```python
from build123d import *

# Parameters (mm, degrees)
SKETCH1_R           = 6.35
SKETCH1_R_2         = 4.699
BOSS_EXTRUDE1_DEPTH = 13.716
SKETCH2_R           = 7.5565
SKETCH2_R_2         = 6.096
BOSS_EXTRUDE2_DEPTH = 1.27
SKETCH3_R           = 6.35
BOSS_EXTRUDE3_DEPTH = 1.016


with BuildPart() as part:
    # Sketch1 → Boss-Extrude1 (new body)
    with BuildSketch(Plane(origin=(0, 0, 0), x_dir=(1, 0, 0), z_dir=(0, 1, 0))):
        Circle(SKETCH1_R)
        Circle(SKETCH1_R_2, mode=Mode.SUBTRACT)
    extrude(amount=BOSS_EXTRUDE1_DEPTH)

    # Sketch2 → Boss-Extrude2 (add)
    with BuildSketch(Plane(origin=(0, 0, 0), x_dir=(1, 0, 0), z_dir=(0, 1, 0))):
        Circle(SKETCH2_R)
        Circle(SKETCH2_R_2, mode=Mode.SUBTRACT)
    extrude(amount=BOSS_EXTRUDE2_DEPTH)

    # Sketch3 → Boss-Extrude3 (add)
    with BuildSketch(Plane(origin=(0, 13.716, 0), x_dir=(1, 0, 0), z_dir=(0, 1, 0))):
        Circle(SKETCH3_R)
    extrude(amount=-BOSS_EXTRUDE3_DEPTH)


solid = part.part
```
Verification items for the finished model (mm, model axes). A direction names the side the tool comes from. Give positions to 0.01 mm unless a question says otherwise; leave off trailing zeros. Order: outer loops, then holes, each group sorted by start corner. A loop starts at its lowest first (then second) coordinate and runs counter-clockwise, first axis right, second up. Notation, with made-up numbers: (46, -22.5) -> (66, -22.5) arc R16 ccw to (66, -4.5) -> close; hole circle Ø10 at (48.5, 8.5). An arc over 180 degrees is marked (long way). One line per item, written item: value.
(1) Gauge pin test, flat ends, axial feed: pin 1 (1.5 mm diameter, centred on x = -4.5, y = 8, fed in from +Z); pin 2 (5.5 mm diameter, centred on x = 0, z = 0, fed in from -Y); pin 3 (2 mm diameter, centred on y = 8.5, z = 1, fed in from +X). Record the tip position at first contact, or that the pin passes through.
Final values:
pin 1: z = 5.12
pin 2: y = 12.7
pin 3: x = 6.35
(2) Sectioned sample at D-D on x = 6. Record the cut outline in (y, z), then the cut area to 3 significant figures.
Final values:
outline: (0, -4.59) -> (1.27, -4.59) -> (1.27, -2.08) -> (13.72, -2.08) -> (13.72, 2.08) -> (1.27, 2.08) -> (1.27, 4.59) -> (0, 4.59) -> close
area: 63.4 mm^2
(3) Scan lines: line 1 along Z through (x, y) = (0, 4.25); line 2 along Y through (x, z) = (-3.25, 1.75). Record each from-to range of solid material in increasing order. Write a range as [from, to].
Final values:
line 1: [-6.35, -4.7], [4.7, 6.35]
line 2: [12.7, 13.72]
(4) Draft check along X on faces 1 (the face through (0, 13.716, 0)), 2 (the face through (0, 12.7, 0)), 3 (the face through (-0.61, 6.26, -4.66)), 4 (the face through (-5.569, 0.626, -5.107)). Enter one of: pulls with the +X half, pulls with the -X half, needs draft (parallel to the pull), parting line crosses it, or undercut.
Final values:
face 1: needs draft
face 2: undercut
face 3: undercut
face 4: parting line crosses it
(5) Sectioned sample at B-B on x = 0. Record the cut outline in (y, z), then the cut area to 3 significant figures.
Final values:
outline: (0, -7.56) -> (1.27, -7.56) -> (1.27, -6.35) -> (13.72, -6.35) -> (13.72, 6.35) -> (1.27, 6.35) -> (1.27, 7.56) -> (0, 7.56) -> (0, 4.7) -> (12.7, 4.7) -> (12.7, -4.7) -> (0, -4.7) -> close
area: 57.9 mm^2
(6) Tool access check on faces 5 (the face through (5, 0, 0)), 6 (the face through (-1.38, 7.41, 6.2)). Record the directions out of +Z, -Z, +X, -X, +Y, -Y that give a thin tool (end or side, any length) a straight path to the whole face; none if there is none.
Final values:
face 5: +Z, -Z, +X, -X, -Y
face 6: +Y
(7) Sectioned sample at C-C on y = 2.75. Record the cut outline in (x, z), then the cut area to 3 significant figures.
Final values:
outline: circle Ø12.7 at (0, 0); hole circle Ø9.4 at (0, 0)
area: 57.3 mm^2
(8) Sectioned sample at A-A on z = 0. Record the cut outline in (x, y).
Final values:
outline: (-7.56, 0) -> (-4.7, 0) -> (-4.7, 12.7) -> (4.7, 12.7) -> (4.7, 0) -> (7.56, 0) -> (7.56, 1.27) -> (6.35, 1.27) -> (6.35, 13.72) -> (-6.35, 13.72) -> (-6.35, 1.27) -> (-7.56, 1.27) -> close
